Design review of the part built by this model. Coordinates are the model's own, in mm. A direction names the side the tool comes from. Round coordinates to 2 decimals unless told otherwise and drop trailing zeros. Write each loop counter-clockwise with the first axis right and the second up, starting at its lowest first coordinate (ties: lowest second). Pieces come first, ordered by that corner, then holes. Notation, with made-up numbers: (-17.75, 70) - (7.25, 70) arc R19 ccw to (7.25, 77) - close; hole circle Ø9 at (15.5, 80.25). An arc over 180 degrees is marked (long way). Use one line per item in the form item = value.
```python
from build123d import *

# Parameters (mm, degrees)
CROQUIS1_W              = 73
CROQUIS1_H              = 69
CROQUIS1_R              = 3.1
CROQUIS1_R_2            = 1.25
SALIENTE_EXTRUIR1_DEPTH = 6
CROQUIS3_W              = 190
CROQUIS3_H              = 120
CROQUIS3_R              = 2.25
CROQUIS3_R_2            = 5
CROQUIS3_R_3            = 1.25
SALIENTE_EXTRUIR2_DEPTH = 3
CROQUIS5_R              = 2.75
CORTAR_EXTRUIR1_DEPTH   = 3


with BuildPart() as part:
    # Croquis1 → Saliente-Extruir1 (new body)
    with BuildSketch(Plane.XY):
        with Locations((36.5, 34.5)):
            Rectangle(CROQUIS1_W, CROQUIS1_H)
        with Locations((6.5, 6.5)):
            Circle(CROQUIS1_R, mode=Mode.SUBTRACT)
        with Locations((66.5, 6.5)):
            Circle(CROQUIS1_R, mode=Mode.SUBTRACT)
        with Locations((66.5, 62.5)):
            Circle(CROQUIS1_R, mode=Mode.SUBTRACT)
        with Locations((6.5, 62.5)):
            Circle(CROQUIS1_R, mode=Mode.SUBTRACT)
        with Locations((18.5, 50.5)):
            Circle(CROQUIS1_R_2, mode=Mode.SUBTRACT)
        with Locations((54.5, 50.5)):
            Circle(CROQUIS1_R_2, mode=Mode.SUBTRACT)
        with Locations((54.5, 18.5)):
            Circle(CROQUIS1_R_2, mode=Mode.SUBTRACT)
        with Locations((18.5, 18.5)):
            Circle(CROQUIS1_R_2, mode=Mode.SUBTRACT)
    extrude(amount=SALIENTE_EXTRUIR1_DEPTH)

    # Croquis3 → Saliente-Extruir2 (add)
    with BuildSketch(Plane(origin=(0, 0, 0), x_dir=(-1, 0, 0), z_dir=(0, 0, -1))):
        with Locations((-34.5, 32.5)):
            Rectangle(CROQUIS3_W, CROQUIS3_H)
        with Locations((36.5, 32.5)):
            Circle(CROQUIS3_R, mode=Mode.SUBTRACT)
        with Locations((-91.623199077, 0.069259856)):
            Circle(CROQUIS3_R, mode=Mode.SUBTRACT)
        with Locations((-91.623199077, 64.930740144)):
            Circle(CROQUIS3_R, mode=Mode.SUBTRACT)
        with Locations((-66.5, 62.5)):
            Circle(CROQUIS3_R_2, mode=Mode.SUBTRACT)
        with Locations((-6.5, 62.5)):
            Circle(CROQUIS3_R_2, mode=Mode.SUBTRACT)
        with Locations((-6.5, 6.5)):
            Circle(CROQUIS3_R_2, mode=Mode.SUBTRACT)
        with Locations((-66.5, 6.5)):
            Circle(CROQUIS3_R_2, mode=Mode.SUBTRACT)
        with Locations((-54.5, 50.5)):
            Circle(CROQUIS3_R_3, mode=Mode.SUBTRACT)
        with Locations((-18.5, 50.5)):
            Circle(CROQUIS3_R_3, mode=Mode.SUBTRACT)
        with Locations((-18.5, 18.5)):
            Circle(CROQUIS3_R_3, mode=Mode.SUBTRACT)
        with Locations((-54.5, 18.5)):
            Circle(CROQUIS3_R_3, mode=Mode.SUBTRACT)
    extrude(amount=SALIENTE_EXTRUIR2_DEPTH)

    # Croquis5 → Cortar-Extruir1 (cut)
    with BuildSketch(Plane.XY.offset(6)):
        with Locations((18.5, 50.5)):
            Circle(CROQUIS5_R)
        with Locations((54.5, 50.5)):
            Circle(CROQUIS5_R)
        with Locations((54.5, 18.5)):
            Circle(CROQUIS5_R)
        with Locations((18.5, 18.5)):
            Circle(CROQUIS5_R)
    extrude(amount=-CORTAR_EXTRUIR1_DEPTH, mode=Mode.SUBTRACT)


solid = part.part
```
Q1. We need section B-B on z = -1.5. State how many separate pieces and enclosed holes the cut face has, then the cut area to 3 significant figures.
Calculated:
separate_pieces = 1
enclosed_holes = 11
area = 22,400 mm2
Q2. We need section D-D on x = -3. Write out the cut boundary in (y, z).
Calculated:
outline = (-27.5, -3) - (92.5, -3) - (92.5, 0) - (-27.5, 0) - close
Q3. For P1, Ø5, axis at x = 18.5, y = 50.5, coming from the +Z side; P2, Ø2, axis at x = 52.5, y = -11.5, coming from the +Z side; P3, Ø7, axis at x = 6.5, y = 6.5, coming from the -Z side, all flat-tipped, find the tip position at first contact; note any pin that passes through.
Calculated:
P1 = 3
P2 = 0
P3 = 0
Q4. We need section A-A on y = 32.5. Write out the cut boundary in (x, z).
Calculated:
outline = (-60.5, -3) - (-38.75, -3) - (-38.75, 0) - (-60.5, 0) - close; (-34.25, -3) - (129.5, -3) - (129.5, 0) - (73, 0) - (73, 6) - (0, 6) - (0, 0) - (-34.25, 0) - close
Q5. To check wall thickness, follow line 1 along X through (y, z) = (18.5, 1.25); line 2 along Y through (x, z) = (18.5, -1.4); line 3 along X through (y, z) = (18.5, -1.6). State the ranges of each line that lie inside material, in increasing order. Write a range as from..to.
Calculated:
line_1 = 0..17.25, 19.75..53.25, 55.75..73
line_2 = -27.5..17.25, 19.75..49.25, 51.75..92.5
line_3 = -60.5..17.25, 19.75..53.25, 55.75..129.5
Q6. Draft analysis for pull direction Y (two halves, no side actions). For faces 1 (the flat face through (36, 0, 3)), 2 (the flat face through (36, 33, -3)), 3 (the cylindrical face through (4.04, 4.614, 2.958)), state which applies: released by +Y, released by -Y, zero draft, split by the parting line, or undercut.
Calculated:
face_1 = released by -Y
face_2 = zero draft
face_3 = undercut
Q7. Machinability: for faces 4 (the flat face through (9, 9, 0)), 5 (the cylindrical face through (-37.71, 34.397, -1.479)), 6 (the cylindrical face through (18.142, 53.227, 4.521)), which of the approach directions +Z, -Z, +X, -X, +Y, -Y give a long, thin tool a straight path to every point of the face, cutting with its end or side? Answer none if there is none.
Calculated:
face_4 = -Z
face_5 = +Z, -Z
face_6 = +Z
Q8. We need section C-C on y = 80. Write out the cut boundary in (x, z), then the cut area to 3 significant figures.
Calculated:
outline = (-60.5, -3) - (129.5, -3) - (129.5, 0) - (-60.5, 0) - close
area = 570 mm2
